from build123d import *

# Parameters (mm, degrees)
SKETCH_1_W          = 40
SKETCH_1_H          = 100
SKETCH_1_R          = 1.6
SKETCH_1_R_2        = 3
EXTRUDE_1_DEPTH     = 3
SKETCH_2_W          = 20
SKETCH_2_H          = 20
CUT_EXTRUDE_1_DEPTH = 108.745069493
SKETCH_3_W          = 20
SKETCH_3_H          = 40
CUT_EXTRUDE_2_DEPTH = 10
CHAMFER_1_SIZE      = 3


with BuildPart() as part:
    # ｽｹｯﾁ1 → ﾎﾞｽ - 押し出し1 (new body)
    with BuildSketch(Plane.XY):
        with Locations((20, 50)):
            Rectangle(SKETCH_1_W, SKETCH_1_H)
        with Locations((5, 95)):
            Circle(SKETCH_1_R, mode=Mode.SUBTRACT)
        with Locations((35, 95)):
            Circle(SKETCH_1_R, mode=Mode.SUBTRACT)
        with Locations((5, 80)):
            Circle(SKETCH_1_R_2, mode=Mode.SUBTRACT)
        with Locations((35, 70)):
            Circle(SKETCH_1_R_2, mode=Mode.SUBTRACT)
        with Locations((5, 20)):
            Circle(SKETCH_1_R_2, mode=Mode.SUBTRACT)
        with Locations((35, 30)):
            Circle(SKETCH_1_R_2, mode=Mode.SUBTRACT)
        with Locations((5, 5)):
            Circle(SKETCH_1_R, mode=Mode.SUBTRACT)
        with Locations((35, 5)):
            Circle(SKETCH_1_R, mode=Mode.SUBTRACT)
    extrude(amount=EXTRUDE_1_DEPTH)

    # ｽｹｯﾁ2 → ｶｯﾄ - 押し出し1 (cut, through all)
    with BuildSketch(Plane.XY.offset(3)):
        with Locations((20, 90)):
            Rectangle(SKETCH_2_W, SKETCH_2_H)
        with Locations((20, 10)):
            Rectangle(SKETCH_2_W, SKETCH_2_H)
    extrude(amount=-CUT_EXTRUDE_1_DEPTH, mode=Mode.SUBTRACT)

    # ｽｹｯﾁ3 → ｶｯﾄ - 押し出し2 (cut)
    with BuildSketch(Plane.XY.offset(3)):
        with Locations((20, 50)):
            Rectangle(SKETCH_3_W, SKETCH_3_H)
    extrude(amount=-CUT_EXTRUDE_2_DEPTH, mode=Mode.SUBTRACT)

    # 面取り1
    chamfer_1_edges = [part.edges().sort_by_distance(p)[0] for p in [
        (10, 80, 1.5),
        (30, 80, 1.5),
        (10, 20, 1.5),
        (30, 20, 1.5),
        (30, 70, 1.5),
        (30, 30, 1.5),
        (10, 30, 1.5),
        (10, 70, 1.5),
    ]]
    chamfer(chamfer_1_edges, length=CHAMFER_1_SIZE)


solid = part.part
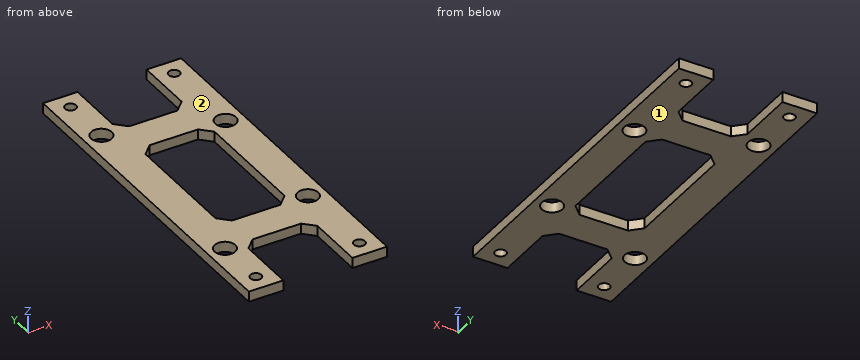
Can you work these out from the model? Positions are in its coordinate system, mm. Face numbers are marked on the shaded views. Give positions to 0.01 mm unless a question says otherwise; leave off trailing zeros. Order: outer loops, then holes, each group sorted by start corner. A loop starts at its lowest first (then second) coordinate and runs counter-clockwise, first axis right, second up. Notation, with made-up numbers: (1.5, 43.5) - (20.5, 43.5) arc R26 ccw to (20.5, 68.5) - close; hole circle Ø10 at (-19, 66). An arc over 180 degrees is marked (long way). Write each question's results on one line, items separated by ' | '.
1) If we mould it in two halves opening along Z, with no side actions, what happens to the marked faces 1 and 2? For each: pulls with the +Z half, pulls with the -Z half, needs draft (parallel to the pull), parting line crosses it, or undercut.
Final values:
face 1: pulls with the -Z half | face 2: pulls with the +Z half
2) Suppose I cut it at B-B, the plane y = 5. Write out the boundary of the cut face in (x, z), then the cut area to 3 significant figures.
Final values:
outline: (0, 0) - (3.4, 0) - (3.4, 3) - (0, 3) - close; (6.6, 0) - (10, 0) - (10, 3) - (6.6, 3) - close; (30, 0) - (33.4, 0) - (33.4, 3) - (30, 3) - close; (36.6, 0) - (40, 0) - (40, 3) - (36.6, 3) - close | area: 40.8 mm^2
3) Please list where these lines run through material, in increasing order: line 1 along X through (y, z) = (95, 1.4); line 2 along Y through (x, z) = (35, 2.35); line 3 along X through (y, z) = (66, 0.9). Write a range as [from, to].
Final values:
line 1: x = [0, 3.4], [6.6, 10], [30, 33.4], [36.6, 40] | line 2: y = [0, 3.4], [6.6, 27], [33, 67], [73, 93.4], [96.6, 100] | line 3: x = [0, 10], [30, 40]
4) Suppose I cut it at D-D, the plane x = 35. Write out the boundary of the cut face in (y, z), then the cut area to 3 significant figures.
Final values:
outline: (0, 0) - (3.4, 0) - (3.4, 3) - (0, 3) - close; (6.6, 0) - (27, 0) - (27, 3) - (6.6, 3) - close; (33, 0) - (67, 0) - (67, 3) - (33, 3) - close; (73, 0) - (93.4, 0) - (93.4, 3) - (73, 3) - close; (96.6, 0) - (100, 0) - (100, 3) - (96.6, 3) - close | area: 245 mm^2
5) Suppose I cut it at C-C, the plane z = 2.2. Give the number of separate pieces and of enclosed holes in the cut face, then the cut area to 3 significant figures.
Final values:
separate pieces: 1 | enclosed holes: 9 | area: 2,290 mm^2
6) I'm going to push flat-ended pins straight in: pin 1 Ø3.5 at (x, y) = (35, 30) entering from -Z; pin 2 Ø1.5 at (x, z) = (11.5, 2) entering from +Y; pin 3 Ø1.5 at (x, z) = (17.5, 2) entering from -Y; pin 4 Ø1.5 at (x, z) = (22.5, 2) entering from +Y. Where does each tip first touch, or does it pass through?
Final values:
pin 1: passes through | pin 2: stops at y = 82.25 | pin 3: stops at y = 20 | pin 4: stops at y = 80
7) Suppose I cut it at A-A, the plane x = 23.5. Write out the boundary of the cut face in (y, z).
Final values:
outline: (20, 0) - (30, 0) - (30, 3) - (20, 3) - close; (70, 0) - (80, 0) - (80, 3) - (70, 3) - close
